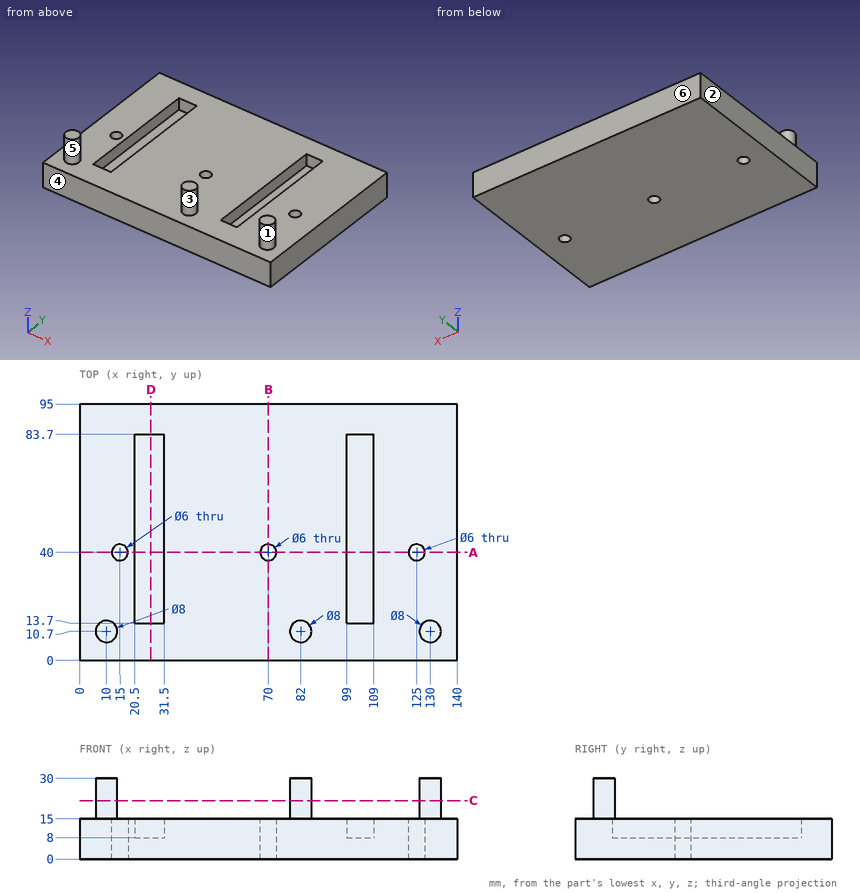
Design review of the part shown in the three views and the two pictorial views. Dimensions are in mm from the part's minimum x, y and z. A direction names the side the tool comes from. Coordinates: 2 decimals unless noted, no trailing zeros. Write each loop counter-clockwise with the first axis right and the second up, starting at its lowest first coordinate (ties: lowest second). Pieces come first, ordered by that corner, then holes.
(1) Wall thickness on probe 1 along X at (y, z) = (40, 7.25); probe 2 along X at (y, z) = (52.5, 14.5); probe 3 along Y at (x, z) = (125, 4): over which ranges is each line inside the solid? List them lowest first.
(2) The part is to be moulded in two halves that separate along X. For the marked faces 1, 2, 3 and 4, say which applies: +X half, -X half, draft (parallel to the pull), parting line (faces both ways), or undercut.
(3) Add section C-C on z = 21.75. Give the boundary of the cut face in (x, y), then the cut area to 3 significant figures.
(4) Add section D-D on x = 26.5. Give the boundary of the cut face in (y, z).
(5) Tool access review of the marked faces 5 and 6: name each direction out of +Z, -Z, +X, -X, +Y, -Y from which nothing blocks a thin tool from reaching the whole face with its end or side.
(6) Add section A-A on y = 40. Give the boundary of the cut face in (x, z).
(7) Add section B-B on x = 70. Give the boundary of the cut face in (y, z).
(8) For pin 1 Ø3 at (x, y) = (102, 46) entering from +Z; pin 2 Ø2 at (x, y) = (42, 23.5) entering from +Z, all flat-tipped, find the tip position at first contact; note any pin that passes through.
Answer sheet:
1. probe 1: x = 0 to 12, 18 to 67, 73 to 122, 128 to 140
1. probe 2: x = 0 to 20.5, 31.5 to 99, 109 to 140
1. probe 3: y = 0 to 37, 43 to 95
2. face 1: undercut
2. face 2: -X half
2. face 3: undercut
2. face 4: draft
3. outline: circle Ø8 at (10, 10.7); circle Ø8 at (82, 10.7); circle Ø8 at (130, 10.7)
3. area: 151 mm2
4. outline: (0, 0) - (95, 0) - (95, 15) - (83.7, 15) - (83.7, 8) - (13.7, 8) - (13.7, 15) - (0, 15) - close
5. face 5: +Z
5. face 6: +Z, -Z, +X, -X, +Y
6. outline: (0, 0) - (12, 0) - (12, 15) - (0, 15) - close; (18, 0) - (67, 0) - (67, 15) - (31.5, 15) - (31.5, 8) - (20.5, 8) - (20.5, 15) - (18, 15) - close; (73, 0) - (122, 0) - (122, 15) - (109, 15) - (109, 8) - (99, 8) - (99, 15) - (73, 15) - close; (128, 0) - (140, 0) - (140, 15) - (128, 15) - close
7. outline: (0, 0) - (37, 0) - (37, 15) - (0, 15) - close; (43, 0) - (95, 0) - (95, 15) - (43, 15) - close
8. pin 1: stops at z = 8
8. pin 2: stops at z = 15
